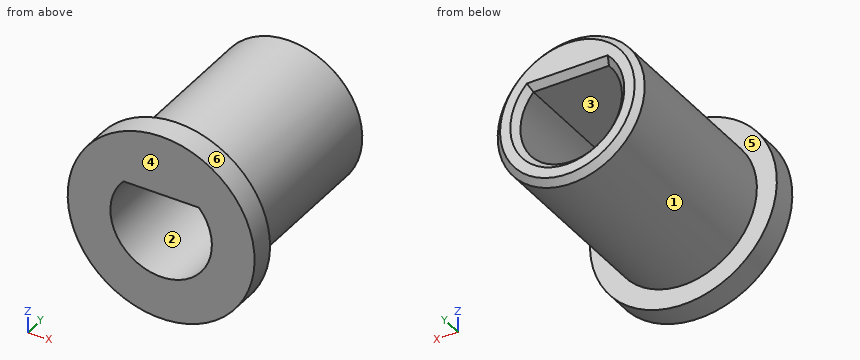
```python
from build123d import *

# Parameters (mm, degrees)
SCHNITT_LINEAR_AUSTRAGEN1_DEPTH = 21.03746491
FASE1_SIZE                      = 0.5


with BuildPart() as part:
    # Skizze1 → Rotation1 (revolve)
    with BuildSketch(Plane.XY, mode=Mode.PRIVATE) as rotation1_sk:
        Polygon((0, 0), (7.5, 0), (7.5, 2), (5.9, 2), (5.9, 17), (0, 17), align=None)
    revolve(rotation1_sk.sketch.rotate(Axis((0, 0, 0), (0, -1, 0)), 90), axis=Axis((0, 0, 0), (0, -1, 0)))

    # Skizze2 → Schnitt-Linear austragen1 (cut, through all)
    with BuildSketch(Plane(origin=(0, 17, 0), x_dir=(1, 0, 0), z_dir=(0, 1, 0))):
        with BuildLine():
            Line((-3.029851482, -2.725), (3.029851482, -2.725))
            ThreePointArc((3.029851482, -2.725), (0, 4.075), (-3.029851482, -2.725))
        make_face()
    extrude(amount=-SCHNITT_LINEAR_AUSTRAGEN1_DEPTH, mode=Mode.SUBTRACT)

    # Fase1
    fase1_edges = [part.edges().sort_by_distance(p)[0] for p in [
        (0, 17, -4.075),
        (0, 17, 2.725),
        (0, 17, -5.9),
    ]]
    chamfer(fase1_edges, length=FASE1_SIZE)


solid = part.part
```
Source: CAD feature listing. Evaluate the final solid. Frame: model axes, mm. Face numbers are marked on the shaded views. A direction names the side the tool comes from. Give positions to 0.01 mm unless a question says otherwise; leave off trailing zeros. Loops run counter-clockwise (first coordinate to the right, second up) from the corner with the lowest first, then second, coordinate; pieces in that order, holes last. Notation, with made-up numbers: M 69.25,-9.75 L 86.25,-9.75 A31 cw 86.25,27.25 Z; hole C -20.5,83 d5. An arc over 180 degrees is marked long. Put each result on its own line as item: value.
Q1. Section B-B (z = 0). Return the cut outline in (x, y) (3 decimals).
Response values:
outline: M -7.5,0 L -4.075,0 L -4.075,16.5 L -4.575,17 L -5.4,17 L -5.9,16.5 L -5.9,2 L -7.5,2 Z; M 4.075,0 L 7.5,0 L 7.5,2 L 5.9,2 L 5.9,16.5 L 5.4,17 L 4.575,17 L 4.075,16.5 Z
Q2. Line query: probe 1 along X at (y, z) = (11, 0) (3 decimals); probe 2 along Z at (x, y) = (3.25, 6); probe 3 along X at (y, z) = (11.25, -3.5). Output: solid intervals per line, ascending. Write a range as [from, to].
Response values:
probe 1: x = [-5.9, -4.075], [4.075, 5.9]
probe 2: z = [-4.92, -2.46], [2.46, 4.92]
probe 3: x = [-4.75, -2.09], [2.09, 4.75]
Q3. Section C-C (y = 15.25). Return the cut outline in (x, z) (3 decimals), and give its area (3 significant figures).
Response values:
outline: C 0,0 d11.8; hole M -3.03,2.725 A4.075 ccw long 3.03,2.725 Z
area: 62.9 mm²
Q4. Reachability of the marked faces 5 and 6 from +Z, -Z, +X, -X, +Y, -Y: full face, straight path, thin tool, end or side. Return the list, or none.
Response values:
face 5: +Y
face 6: +Y, -Y
Q5. Section A-A (x = 0). Return the cut outline in (y, z) (3 decimals).
Response values:
outline: M 0,-7.5 L 2,-7.5 L 2,-5.9 L 16.5,-5.9 L 17,-5.4 L 17,-4.575 L 16.5,-4.075 L 0,-4.075 Z; M 0,2.725 L 16.5,2.725 L 17,3.225 L 17,5.4 L 16.5,5.9 L 2,5.9 L 2,7.5 L 0,7.5 Z
Q6. Mould query, pull axis Z, two halves, no side actions, for the marked faces 1, 2, 3 and 4. Classes: released by +Z, released by -Z, zero draft, split by the parting line, or undercut.
Response values:
face 1: split by the parting line
face 2: undercut
face 3: undercut
face 4: zero draft
Q7. Pin query (flat end, axial travel): P1, Ø1.5, axis at x = 1, z = 3, coming from the -Y side; P2, Ø1.5, axis at y = 3, z = 0, coming from the -X side; P3, Ø5, axis at x = 0, z = 0, coming from the +Y side; P4, Ø1.5, axis at y = 2, z = -4.5, coming from the +X side. Return the tip coordinate at first contact, or that it passes through.
Response values:
P1: stops at y = 0
P2: stops at x = -5.9
P3: passes through
P4: stops at x = 6.5
